Work out the finished part from the listing and answer in its coordinate system (mm). A direction names the side the tool comes from. Round coordinates to 2 decimals unless told otherwise and drop trailing zeros. Loops run counter-clockwise (first coordinate to the right, second up) from the corner with the lowest first, then second, coordinate; pieces in that order, holes last. Notation, with made-up numbers: (43, -17.75) -> (64, -17.75) arc R29 cw to (64, 10.25) -> close; hole circle Ø5 at (64.25, -26.75). An arc over 180 degrees is marked (long way). Use one line per item in the form item = value.
```python
from build123d import *

# Parameters (mm, degrees)
SKETCH1_R           = 2.38125
BOSS_EXTRUDE1_DEPTH = 228.6
SKETCH2_W           = 6.35
SKETCH2_H           = 38.1
BOSS_EXTRUDE2_DEPTH = 6.35
SKETCH3_R           = 3.175
BOSS_EXTRUDE3_DEPTH = 50.8


with BuildPart() as part:
    # Sketch1 → Boss-Extrude1 (new body)
    with BuildSketch(Plane.XY):
        Circle(SKETCH1_R)
    extrude(amount=BOSS_EXTRUDE1_DEPTH)

    # Sketch2 → Boss-Extrude2 (add)
    with BuildSketch(Plane.XY.offset(228.6)):
        with Locations((0.040964163, 15.489894183)):
            Rectangle(SKETCH2_W, SKETCH2_H)
    extrude(amount=BOSS_EXTRUDE2_DEPTH)

    # Sketch3 → Boss-Extrude3 (add)
    with BuildSketch(Plane.XY.offset(234.95)):
        with Locations((0.040964163, 31.442054565)):
            Circle(SKETCH3_R)
    extrude(amount=BOSS_EXTRUDE3_DEPTH)


solid = part.part
```
(1) Find section B-B, the plane z = 90. Write down the section's boundary in (x, y).
Completed:
outline = circle Ø4.76 at (0, 0)
(2) Find section A-A, the plane y = 0. Write down the section's boundary in (x, z).
Completed:
outline = (-3.13, 228.6) -> (-2.38, 228.6) -> (-2.38, 0) -> (2.38, 0) -> (2.38, 228.6) -> (3.22, 228.6) -> (3.22, 234.95) -> (-3.13, 234.95) -> close
(3) For faces 1 (the cylindrical face through (1.506, 28.625, 259.994)), 2 (the cylindrical face through (-1.89, -1.45, 112.7)), 3 (the flat face through (-3.134, 15, 232)), determine the directions among +Z, -Z, +X, -X, +Y, -Y from which every point of the face is accessible in a straight line to the end or side of a thin tool.
Completed:
face_1 = +Z
face_2 = -Z
face_3 = +Z, -Z, -X, +Y, -Y
(4) Find section C-C, the plane y = 11. Write down the section's boundary in (x, z), then the cut area to 3 significant figures.
Completed:
outline = (-3.13, 228.6) -> (3.22, 228.6) -> (3.22, 234.95) -> (-3.13, 234.95) -> close
area = 40.3 mm2
(5) Consider L1, parallel to Y at x = -0.25, z = 131.5; L2, parallel to Z at x = 1, y = 20.5; L3, parallel to Y at x = 0.5, z = 236.5. Determine where each line is inside the solid, lowest interval first.
Completed:
L1 = -2.37 to 2.37
L2 = 228.6 to 234.95
L3 = 28.3 to 34.58
(6) Given P1, Ø1, axis at x = -1.5, z = 92, coming from the -Y side; P2, Ø1.9, axis at x = -0.5, z = 232.5, coming from the +Y side; P3, Ø5, axis at y = 6, z = 122.5, coming from the -X side; P4, Ø1.9, axis at x = -0.5, y = 24.5, coming from the -Z side, each flat-ended and moving along its own axis, determine where each tip first touches the part or whether it passes through.
Completed:
P1 = -2.16
P2 = 34.54
P3 = through
P4 = 228.6
